Input: part model. Units: mm. Frame: model coordinates. A direction names the side the tool comes from. Round coordinates to 2 decimals unless told otherwise and drop trailing zeros. Write each loop counter-clockwise with the first axis right and the second up, starting at its lowest first coordinate (ties: lowest second). Pieces come first, ordered by that corner, then holes. Notation, with made-up numbers: (-29, -28.5) -> (22, -28.5) arc R30 cw to (22, 9.5) -> close; hole circle Ø6 at (-2.5, 70). An arc over 180 degrees is marked (long way). Write item = value, one per line.
```python
from build123d import *

# Parameters (mm, degrees)
CUT_EXTRUDE2_REACH     = 47.048
SKETCH3_R              = 2.6
CUT_EXTRUDE3_REACH     = 50.063
M6_TAPPED_HOLE2_REACH  = 56.337
M6_TAPPED_HOLE2_BORE_R = 2.5


with BuildPart() as part:
    # Sketch1 → Revolve1 (revolve)
    with BuildSketch(Plane(origin=(0, 0, 0), x_dir=(0, 0, -1), z_dir=(1, 0, 0)), mode=Mode.PRIVATE) as revolve1_sk:
        Polygon((6, 0), (28.4, 0), (28.4, 6), (15, 6), (15, 26.4), (6, 26.4), align=None)
    revolve(revolve1_sk.sketch.rotate(Axis((0, 21.767139862, 0), (0, -1, 0)), 180), axis=Axis((0, 21.767139862, 0), (0, -1, 0)))

    # Sketch3 → Cut-Extrude2 (cut, up to next)
    with BuildSketch(Plane(origin=(0, 6, 0), x_dir=(1, 0, 0), z_dir=(0, 1, 0)), mode=Mode.PRIVATE) as cut_extrude2_sk1:
        with Locations(Location((-22.5, 0, 0), (0, 0, 270))):
            Circle(SKETCH3_R)
    cut_extrude2_tool1 = extrude(cut_extrude2_sk1.sketch, amount=-CUT_EXTRUDE2_REACH, mode=Mode.PRIVATE) & part.part
    # Sketch3 → Cut-Extrude2 (cut, up to next)
    with BuildSketch(Plane(origin=(0, 6, 0), x_dir=(1, 0, 0), z_dir=(0, 1, 0)), mode=Mode.PRIVATE) as cut_extrude2_sk2:
        with Locations(Location((11.25, 19.485571585, 0), (0, 0, 270))):
            Circle(SKETCH3_R)
    cut_extrude2_tool2 = extrude(cut_extrude2_sk2.sketch, amount=-CUT_EXTRUDE2_REACH, mode=Mode.PRIVATE) & part.part
    # Sketch3 → Cut-Extrude2 (cut, up to next)
    with BuildSketch(Plane(origin=(0, 6, 0), x_dir=(1, 0, 0), z_dir=(0, 1, 0)), mode=Mode.PRIVATE) as cut_extrude2_sk3:
        with Locations(Location((11.25, -19.485571585, 0), (0, 0, 270))):
            Circle(SKETCH3_R)
    cut_extrude2_tool3 = extrude(cut_extrude2_sk3.sketch, amount=-CUT_EXTRUDE2_REACH, mode=Mode.PRIVATE) & part.part
    # Sketch3 → Cut-Extrude2 (cut, up to next)
    with BuildSketch(Plane(origin=(0, 6, 0), x_dir=(1, 0, 0), z_dir=(0, 1, 0)), mode=Mode.PRIVATE) as cut_extrude2_sk4:
        with Locations(Location((23.75, 0, 0), (0, 0, 270))):
            Circle(SKETCH3_R)
    cut_extrude2_tool4 = extrude(cut_extrude2_sk4.sketch, amount=-CUT_EXTRUDE2_REACH, mode=Mode.PRIVATE) & part.part
    # Sketch3 → Cut-Extrude2 (cut, up to next)
    with BuildSketch(Plane(origin=(0, 6, 0), x_dir=(1, 0, 0), z_dir=(0, 1, 0)), mode=Mode.PRIVATE) as cut_extrude2_sk5:
        with Locations(Location((-11.875, -20.56810334, 0), (0, 0, 270))):
            Circle(SKETCH3_R)
    cut_extrude2_tool5 = extrude(cut_extrude2_sk5.sketch, amount=-CUT_EXTRUDE2_REACH, mode=Mode.PRIVATE) & part.part
    # Sketch3 → Cut-Extrude2 (cut, up to next)
    with BuildSketch(Plane(origin=(0, 6, 0), x_dir=(1, 0, 0), z_dir=(0, 1, 0)), mode=Mode.PRIVATE) as cut_extrude2_sk6:
        with Locations(Location((-11.875, 20.56810334, 0), (0, 0, 270))):
            Circle(SKETCH3_R)
    cut_extrude2_tool6 = extrude(cut_extrude2_sk6.sketch, amount=-CUT_EXTRUDE2_REACH, mode=Mode.PRIVATE) & part.part
    add(cut_extrude2_tool1.solids().sort_by_distance((-22.5, 6, 0))[0], mode=Mode.SUBTRACT)
    add(cut_extrude2_tool2.solids().sort_by_distance((11.25, 6, -19.485572))[0], mode=Mode.SUBTRACT)
    add(cut_extrude2_tool3.solids().sort_by_distance((11.25, 6, 19.485572))[0], mode=Mode.SUBTRACT)
    add(cut_extrude2_tool4.solids().sort_by_distance((23.75, 6, 0))[0], mode=Mode.SUBTRACT)
    add(cut_extrude2_tool5.solids().sort_by_distance((-11.875, 6, 20.568103))[0], mode=Mode.SUBTRACT)
    add(cut_extrude2_tool6.solids().sort_by_distance((-11.875, 6, -20.568103))[0], mode=Mode.SUBTRACT)

    # Sketch4 → Cut-Extrude3 (cut, up to next)
    with BuildSketch(Plane(origin=(0, 26.4, 0), x_dir=(1, 0, 0), z_dir=(0, 1, 0)), mode=Mode.PRIVATE) as cut_extrude3_sk1:
        with BuildLine():
            Line((-2, 7.6), (-2, 5.656854249))
            ThreePointArc((-2, 5.656854249), (0, 6), (2, 5.656854249))
            Line((2, 5.656854249), (2, 7.6))
            Line((2, 7.6), (-2, 7.6))
        make_face()
    cut_extrude3_tool1 = extrude(cut_extrude3_sk1.sketch, amount=-CUT_EXTRUDE3_REACH, mode=Mode.PRIVATE) & part.part
    add(cut_extrude3_tool1.solids().sort_by_distance((0, 26.4, -6.740451))[0], mode=Mode.SUBTRACT)

    # M6 Tapped Hole2 bore (on position points) → M6 Tapped Hole2 (cut, up to next)
    with BuildSketch(Plane(origin=(0, 16.2, 15), x_dir=(1, 0, 0), z_dir=(0, 0, 1)), mode=Mode.PRIVATE) as m6_tapped_hole2_sk1:
        Circle(M6_TAPPED_HOLE2_BORE_R)
    m6_tapped_hole2_tool1 = extrude(m6_tapped_hole2_sk1.sketch, amount=-M6_TAPPED_HOLE2_REACH, mode=Mode.PRIVATE) & part.part
    add(m6_tapped_hole2_tool1.solids().sort_by_distance((0, 16.2, 15))[0], mode=Mode.SUBTRACT)


solid = part.part
```
1) Line query: L1, parallel to X at y = 1.7, z = 0; L2, parallel to Z at x = 0, y = 13.5; L3, parallel to Y at x = 14, z = -5.5. Output: solid intervals per line, ascending. Write a range as from..to.
Solutions:
L1 = -28.4..-25.1, -19.9..-6, 6..21.15, 26.35..28.4
L2 = -15..-7.6, 6..15
L3 = 0..6
2) Draft query along Z for faces 5 (the face through (-0.2, 26.4, 6.5)), 6 (the face through (-2, 13, -7)), 7 (the face through (-28.158, 3.042, -3.697)). Return one class per face: +Z half, -Z half, draft (parallel to the pull), parting line (faces both ways), or undercut.
Solutions:
face_5 = draft
face_6 = undercut
face_7 = parting line
3) Cut plane D-D (x = -22.5). Return the cut outline in (y, z), and give its area (3 significant figures).
Solutions:
outline = (0, -17.33) -> (6, -17.33) -> (6, -2.6) -> (0, -2.6) -> close; (0, 2.6) -> (6, 2.6) -> (6, 17.33) -> (0, 17.33) -> close
area = 177 mm^2
4) Access query for faces 1 (the face through (-12.65, 16.34, 8.06)), 2 (the face through (-0.54, 13.76, 10.29)), 3 (the face through (2, 13, -7)), 4 (the face through (-7, 0, 0)). Directions: +Z, -Z, +X, -X, +Y, -Y. A direction counts if a zero-diameter tool reaches every point of the face in a straight line with its end or side. Return the directions, or none.
Solutions:
face_1 = +Y
face_2 = +Z
face_3 = +Y, -Y
face_4 = +Z, -Z, +X, -X, -Y
5) Cut plane B-B (y = 24.25). Return the cut outline in (x, z), and give its area (3 significant figures).
Solutions:
outline = circle Ø30 at (0, 0); hole (-2, -7.6) -> (2, -7.6) -> (2, -5.66) arc R6 ccw (long way) to (-2, -5.66) -> close
area = 587 mm^2
6) First-contact query: P1, Ø1.5, axis at x = 14.5, y = 7.5, coming from the +Z side; P2, Ø6, axis at y = 4, z = 13.5, coming from the -X side; P3, Ø4.5, axis at x = -1, y = 19, coming from the +Z side. Flat tips, straight axial feed; report the tip coordinate or a pass-through.
Solutions:
P1 = 5.99
P2 = -26.39
P3 = 15
7) Cut plane A-A (z = 0). Return the cut outline in (x, y), and give its area (3 significant figures).
Solutions:
outline = (-28.4, 0) -> (-25.1, 0) -> (-25.1, 6) -> (-28.4, 6) -> close; (-19.9, 0) -> (-6, 0) -> (-6, 26.4) -> (-15, 26.4) -> (-15, 6) -> (-19.9, 6) -> close; (6, 0) -> (21.15, 0) -> (21.15, 6) -> (15, 6) -> (15, 26.4) -> (6, 26.4) -> close; (26.35, 0) -> (28.4, 0) -> (28.4, 6) -> (26.35, 6) -> close
area = 574 mm^2
8) Cut plane C-C (x = -10). Return the cut outline in (y, z), and give its area (3 significant figures).
Solutions:
outline = (0, -26.58) -> (6, -26.58) -> (6, -22.37) -> (0, -22.37) -> close; (0, -18.77) -> (6, -18.77) -> (6, -11.18) -> (26.4, -11.18) -> (26.4, 11.18) -> (6, 11.18) -> (6, 18.77) -> (0, 18.77) -> close; (0, 22.37) -> (6, 22.37) -> (6, 26.58) -> (0, 26.58) -> close
area = 732 mm^2
